```python
from build123d import *

# Parameters (mm, degrees)
BOSS_EXTRUDE1_DEPTH = 6.35
CUT_EXTRUDE1_REACH  = 14.7
SKETCH2_R           = 9.525


with BuildPart() as part:
    # Sketch1 → Boss-Extrude1 (new body, symmetric)
    with BuildSketch(Plane(origin=(0, 0, 0), x_dir=(0, 0, -1), z_dir=(1, 0, 0))):
        Polygon((0, 0), (50.8, 0), (50.8, 25.4), (609.6, 25.4), (609.6, 254), (0, 254), align=None)
    extrude(amount=BOSS_EXTRUDE1_DEPTH, both=True)

    # Sketch2 → Cut-Extrude1 (cut, up to next)
    with BuildSketch(Plane(origin=(6.35, 0, 0), x_dir=(0, 0, -1), z_dir=(1, 0, 0)), mode=Mode.PRIVATE) as cut_extrude1_sk1:
        with Locations((25.4, 25.4)):
            Circle(SKETCH2_R)
    cut_extrude1_tool1 = extrude(cut_extrude1_sk1.sketch, amount=-CUT_EXTRUDE1_REACH, mode=Mode.PRIVATE) & part.part
    add(cut_extrude1_tool1.solids().sort_by_distance((6.35, 25.4, -25.4))[0], mode=Mode.SUBTRACT)
    # Sketch2 → Cut-Extrude1 (cut, up to next)
    with BuildSketch(Plane(origin=(6.35, 0, 0), x_dir=(0, 0, -1), z_dir=(1, 0, 0)), mode=Mode.PRIVATE) as cut_extrude1_sk2:
        with Locations((330.2, 50.8)):
            Circle(SKETCH2_R)
    cut_extrude1_tool2 = extrude(cut_extrude1_sk2.sketch, amount=-CUT_EXTRUDE1_REACH, mode=Mode.PRIVATE) & part.part
    add(cut_extrude1_tool2.solids().sort_by_distance((6.35, 50.8, -330.2))[0], mode=Mode.SUBTRACT)


solid = part.part
```
Could you check a few things on this model? Use its own coordinates, in mm. A direction names the side the tool comes from. Coordinates: 2 decimals unless noted, no trailing zeros. Write each loop counter-clockwise with the first axis right and the second up, starting at its lowest first coordinate (ties: lowest second). Pieces come first, ordered by that corner, then holes. Notation, with made-up numbers: (51.25, -29.5) -> (99.25, -29.5) arc R24 ccw to (99.25, -0.5) -> close; hole circle Ø5 at (69, -28.5). An arc over 180 degrees is marked (long way). Write item = value, one per line. Start each with the question number.
(1) Will this pin go through, and if not, where does the flat tip stop? pin 1 (3 mm diameter, centred on x = -1.5, z = -405, fed in from -Y).
(2) Which directions (+Z, -Z, +X, -X, +Y, -Y) give clear straight access to the entire face, cutting with the end or side of a thin tool? Please do faces 5 (the face through (0, 0, -25)), 6 (the face through (0, 13, -50.8)).
(3) We'd pull the mould along Y, two halves only. Please class faces 1 (the face through (0, 25.4, -326)), 2 (the face through (0, 254, -309)), 3 (the face through (0.089, 25.819, -15.884)), 4 (the face through (-6.35, 129, -301)): released by +Y, released by -Y, zero draft, split by the parting line, or undercut.
(4) I want a section at C-C (x = -2). Please give me the cut outline in (y, z) (3 decimals), plus the area to 3 significant figures.
(5) I want a section at D-D (z = -81). Please give me the cut outline in (x, y), plus the area to 3 significant figures.
(6) I want a section at A-A (z = -330.2). Please give me the cut outline in (x, y) (3 decimals).
(7) I want a section at B-B (y = 50.8). Please give me the cut outline in (x, z) (3 decimals), plus the area to 3 significant figures.
(8) I need wall thicknesses on line 1 (Y direction, x = -2.5, z = -330.2) (3 decimals); line 2 (Z direction, x = 5.75, y = 50.5); line 3 (Z direction, x = -1.5, y = 20). Which ranges of each line are inside material? Lowest first, please. Write a range as [from, to].
Result set:
q1.pin_1 = 25.4
q2.face_5 = +Z, -Z, +X, -X, -Y
q2.face_6 = -Z, +X, -X, -Y
q3.face_1 = released by -Y
q3.face_2 = released by +Y
q3.face_3 = undercut
q3.face_4 = zero draft
q4.outline = (0, -50.8) -> (25.4, -50.8) -> (25.4, -609.6) -> (254, -609.6) -> (254, 0) -> (0, 0) -> close; hole circle Ø19.05 at (25.4, -25.4); hole circle Ø19.05 at (50.8, -330.2)
q4.area = 140,000 mm2
q5.outline = (-6.35, 25.4) -> (6.35, 25.4) -> (6.35, 254) -> (-6.35, 254) -> close
q5.area = 2,900 mm2
q6.outline = (-6.35, 25.4) -> (6.35, 25.4) -> (6.35, 41.275) -> (-6.35, 41.275) -> close; (-6.35, 60.325) -> (6.35, 60.325) -> (6.35, 254) -> (-6.35, 254) -> close
q7.outline = (-6.35, -609.6) -> (6.35, -609.6) -> (6.35, -339.725) -> (-6.35, -339.725) -> close; (-6.35, -320.675) -> (6.35, -320.675) -> (6.35, 0) -> (-6.35, 0) -> close
q7.area = 7,500 mm2
q8.line_1 = [25.4, 41.275], [60.325, 254]
q8.line_2 = [-609.6, -339.72], [-320.68, 0]
q8.line_3 = [-50.8, -33.25], [-17.55, 0]
